from build123d import *

# Parameters (mm, degrees)
BOSS_EXTRUDE1_DEPTH = 15.875


with BuildPart() as part:
    # Sketch1 → Boss-Extrude1 (new, symmetric)
    with BuildSketch(Plane(origin=(0, 0, 0), x_dir=(0, 0, -1), z_dir=(1, 0, 0))):
        Polygon((0, 34.925), (0, 50.8), (-57.15, 50.8), (-57.15, -50.8), (0, -50.8), (0, -34.925), (-38.1, -34.925), (-38.1, 34.925), align=None)
    extrude(amount=BOSS_EXTRUDE1_DEPTH, both=True)

    # Sketch2 → F (0.257) Diameter Hole1 (revolve, cut)
    with BuildSketch(Plane(origin=(0, 0, 57.15), x_dir=(0, -1, 0), z_dir=(1, 0, 0))):
        Polygon((0, 0), (0, 19.05), (3.556, 19.05), (3.2639, 18.7579), (3.2639, 0.2921), (3.556, 0), align=None)
    revolve(axis=Axis((0, 0, 63.5), (0, 0, -1)), mode=Mode.SUBTRACT)


solid = part.part
Work out the finished part from the listing and answer in its coordinate system (mm). A direction names the side the tool comes from. Round coordinates to 2 decimals unless told otherwise and drop trailing zeros. Write each loop counter-clockwise with the first axis right and the second up, starting at its lowest first coordinate (ties: lowest second). Pieces come first, ordered by that corner, then holes. Notation, with made-up numbers: (-7, 31) -> (24, 31) arc R15 cw to (24, 46) -> close; hole circle Ø2 at (87.25, 57.25). An arc over 180 degrees is marked (long way). Answer as CSV lines item,"result". Start each with the question number.
(1) The part is cut by section C-C, the plane x = 0. Give the vertices of the cut face in (y, z) (3 decimals).
(2) The mould has two halves that part along X. Classify faces 1 (the flat face through (-15.875, 1, 42)), 2 (the cylindrical face through (3.186, 0.708, 47.754)), 3 (the flat face through (15.875, 1, 42)), 4 (the flat face through (0, -34.925, 19)): +X half, -X half, draft (parallel to the pull), parting line (faces both ways), or undercut.
(3) The part is cut by section D-D, the plane x = 12. Give the vertices of the cut face in (y, z) (3 decimals).
(4) The part is cut by section A-A, the plane y = 0. Give the vertices of the cut face in (x, z) (3 decimals), then the cut area to 3 significant figures.
(5) The part is cut by section B-B, the plane z = 19. Give the vertices of the cut face in (x, y) (3 decimals).
(6) A tool of negligible diameter and unlimited length cuts with its end or side. For faces 5 (the flat face through (0, 34.925, 19)), 6 (the flat face through (0, 43, 0)), from which of +Z, -Z, +X, -X, +Y, -Y can it reach the whole face along a straight path? Write none if from no direction.
(7) Find the intervals of material crossed by probe 1 along Y at (x, z) = (-12, 3.5) (3 decimals); probe 2 along X at (y, z) = (0, 45) (3 decimals); probe 3 along Y at (x, z) = (0, 42), in increasing order.
(8) This flat-tipped pin is pushed along its axis until it touches: pin 1 (3 mm diameter, centred on x = 7, y = -26, fed in from -Z). Where does it stop, or does it pass through?
Output values:
1,outline,"(-50.8, 0) -> (-34.925, 0) -> (-34.925, 38.1) -> (-3.556, 38.1) -> (-3.264, 38.392) -> (-3.264, 56.858) -> (-3.556, 57.15) -> (-50.8, 57.15) -> close; (3.264, 38.392) -> (3.556, 38.1) -> (34.925, 38.1) -> (34.925, 0) -> (50.8, 0) -> (50.8, 57.15) -> (3.556, 57.15) -> (3.264, 56.858) -> close"
2,face 1,"-X half"
2,face 2,"undercut"
2,face 3,"+X half"
2,face 4,"draft"
3,outline,"(-50.8, 0) -> (-34.925, 0) -> (-34.925, 38.1) -> (34.925, 38.1) -> (34.925, 0) -> (50.8, 0) -> (50.8, 57.15) -> (-50.8, 57.15) -> close"
4,outline,"(-15.875, 38.1) -> (-3.556, 38.1) -> (-3.264, 38.392) -> (-3.264, 56.858) -> (-3.556, 57.15) -> (-15.875, 57.15) -> close; (3.264, 38.392) -> (3.556, 38.1) -> (15.875, 38.1) -> (15.875, 57.15) -> (3.556, 57.15) -> (3.264, 56.858) -> close"
4,area,"480 mm²"
5,outline,"(-15.875, -50.8) -> (15.875, -50.8) -> (15.875, -34.925) -> (-15.875, -34.925) -> close; (-15.875, 34.925) -> (15.875, 34.925) -> (15.875, 50.8) -> (-15.875, 50.8) -> close"
6,face 5,"-Z, +X, -X"
6,face 6,"-Z, +X, -X, +Y, -Y"
7,probe 1,"y = -50.8 to -34.925, 34.925 to 50.8"
7,probe 2,"x = -15.875 to -3.264, 3.264 to 15.875"
7,probe 3,"y = -50.8 to -3.26, 3.26 to 50.8"
8,pin 1,"stops at z = 38.1"
